Autodesk Inventor part; units mm, degrees
ref_plane "YZ Plane" through (0, 0, 0) normal (1, 0, 0) x (0, 1, 0)
ref_plane "XZ Plane" through (0, 0, 0) normal (0, 1, 0) x (-1, 0, 0)
ref_plane "XY Plane" through (0, 0, 0) normal (0, 0, 1) x (1, 0, 0)
sketch "Sketch1" plane through (0, 0, 0) normal (0, 1, 0) x (-1, 0, 0)
  circle A0 centre (0, 0) radius 20
  circle A1 centre (0, 0) radius 12.7
  circle A2 centre (0, 0) radius 5.2
  dimension "d1" = 40
  dimension "d14" = 25.4
  dimension "d15" = 10.4
extrude "Extrusion1" add sketch "Sketch1" along normal blind 20 contours A0 | A1 | A2
extrude "Extrusion2" cut sketch "Sketch1" along normal blind 11.4 contours A1 | A2
extrude "Extrusion3" cut sketch "Sketch1" along normal blind 30 contours A2
chamfer "Chamfer2" distance 11.4 distance2 7.5 1 edges at (12.7, 11.4, 0) measured on face at (-12.5355, 7.6, -2.0372)
properties part number "5. ring"
The listing builds one solid part. Answer for the finished solid, in the listing's coordinates (mm). Give positions to 0.01 mm unless a question says otherwise; leave off trailing zeros. Loops run counter-clockwise (first coordinate to the right, second up) from the corner with the lowest first, then second, coordinate; pieces in that order, holes last. Notation, with made-up numbers: M 7,67.5 L 28,67.5 A35 ccw 28,104.5 Z; hole C -19,-9 d5. An arc over 180 degrees is marked long. Answer as CSV lines item,"result".
Item 1: The part is cut by section D-D (z = -17). Give the vertices of the cut face in (x, y).
Values follow:
outline,"M -10.54,0 L 10.54,0 L 10.54,20 L -10.54,20 Z"
Item 2: Straight lines are drawn through the part: line 1 along Z through (x, y) = (0, 15.25); line 2 along X through (y, z) = (14.5, -3); line 3 along X through (y, z) = (2.5, 1). For each, find the intervals that lie inside material, in ascending order. Write a range as [from, to].
Values follow:
line 1,"z = [-20, -5.2], [5.2, 20]"
line 2,"x = [-19.77, -4.25], [4.25, 19.77]"
line 3,"x = [-19.97, -11.01], [11.01, 19.97]"
Item 3: The part is cut by section C-C (y = 13.75). Give the vertices of the cut face in (x, z).
Values follow:
outline,"C 0,0 d40; hole C 0,0 d10.4"
Item 4: Given pin 1 Ø8 at (x, y) = (-5.5, 9) entering from +Z; pin 2 Ø5 at (x, z) = (0.5, 2) entering from -Y; pin 3 Ø12 at (y, z) = (13, -14) entering from -X; pin 4 Ø1 at (x, y) = (4.5, 15.5) entering from +Z, each flat-ended and moving along its own axis, determine where each tip first touches the part or whether it passes through.
Values follow:
pin 1,"stops at z = 19.94"
pin 2,"passes through"
pin 3,"stops at x = -18.33"
pin 4,"stops at z = 19.6"
Item 5: The mould has two halves that part along X. Classify faces 1 (the cylindrical face through (4.336, 9.86, 19.524)), 2 (the conical face through (5.16, 9.42, 3.96)), 3 (the flat face through (-13, 0, 0)): released by +X, released by -X, zero draft, split by the parting line, or undercut.
Values follow:
face 1,"split by the parting line"
face 2,"undercut"
face 3,"zero draft"
